Work out the finished part from the listing and answer in its coordinate system (mm). A direction names the side the tool comes from. Give positions to 0.01 mm unless a question says otherwise; leave off trailing zeros. Write each loop counter-clockwise with the first axis right and the second up, starting at its lowest first coordinate (ties: lowest second). Pieces come first, ordered by that corner, then holes. Notation, with made-up numbers: (68, 88) - (99, 88) arc R28 ccw to (99, 127) - close; hole circle Ø2 at (51, 48.25). An arc over 180 degrees is marked (long way). Write item = value, one per line.
from build123d import *

# Parameters (mm, degrees)
PAD046_DEPTH    = 9
CHAMFER016_SIZE = 3
SKETCH088_R     = 0.6
POCKET040_DEPTH = 7
SKETCH089_W     = 60.467484
SKETCH089_H     = 1.984499
PAD047_DEPTH    = 2


with BuildPart() as part:
    # Sketch085 → Pad046 (new body)
    with BuildSketch(Plane.XY.offset(-11)):
        Polygon((-30.27, -16.85), (30.27, -16.85), (30.27, -36.310793), (25.241268, -47.527155), (24.231199, -56.751064), (-24.231199, -56.751064), (-25.241268, -47.527155), (-30.27, -36.310793), align=None)
    extrude(amount=-PAD046_DEPTH)

    # Chamfer016
    chamfer016_edges = [part.edges().sort_by_distance(p)[0] for p in [
        (24.736234, -52.139109, -20),
        (27.755634, -41.918974, -20),
        (30.27, -26.580397, -20),
        (0, -16.85, -20),
        (-30.27, -26.580397, -20),
        (-27.755634, -41.918974, -20),
        (-24.736234, -52.139109, -20),
    ]]
    chamfer(chamfer016_edges, length=CHAMFER016_SIZE)

    # Sketch088 (on Face4 of Chamfer016) → Pocket040 (cut)
    with BuildSketch(Plane.XY.offset(-11)):
        with Locations((-28.523069, -29.038105)):
            Circle(SKETCH088_R)
        with Locations((28.50172, -29.085497)):
            Circle(SKETCH088_R)
        with Locations((20.999411, -47.657658)):
            Circle(SKETCH088_R)
        with Locations((-21.032127, -47.690895)):
            Circle(SKETCH088_R)
        Polygon((-28.906572, -18.901762), (28.906572, -18.901762), (28.906572, -26.491486), (26.18985, -26.491486), (26.18985, -31.415663), (28.906572, -31.415663), (23.726078, -46.130531), (19.745981, -45.128311), (18.640522, -50.078386), (18.640522, -55.110878), (-18.640522, -55.110878), (-18.640522, -50.078386), (-19.745981, -45.128311), (-23.726078, -46.130531), (-28.906572, -31.415663), (-26.18985, -31.415663), (-26.18985, -26.491486), (-28.906572, -26.491486), align=None)
    extrude(amount=-POCKET040_DEPTH, mode=Mode.SUBTRACT)

    # Sketch089 (on Face4 of Pocket040) → Pad047 (join)
    with BuildSketch(Plane.XY.offset(-11)):
        with Locations((0, -17.897196)):
            Rectangle(SKETCH089_W, SKETCH089_H)
    extrude(amount=PAD047_DEPTH)


with BuildPart() as part_1:
    # Body009 placement: moved
    add(part.part.moved(Location((0, 0, -0.2))))


solid = part_1.part
1. A tool of negligible diameter and unlimited length cuts with its end or side. For faces 1 (the flat face through (0, -55.111, -15)), 2 (the flat face through (0, -18.889, -10)), 3 (the flat face through (0, -16.905, -10)), from which of +Z, -Z, +X, -X, +Y, -Y can it reach the whole face along a straight path? Write none if from no direction.
Solution:
face_1 = +Z
face_2 = +Z, +X, -X, -Y
face_3 = +Z, +X, -X, +Y
2. For a pull along Y with two mould halves and no side action, classify faces 4 (the flat face through (28.75, -26.44, -18.72)), 5 (the flat face through (-21.708, -45.622, -14.651)), 6 (the flat face through (0, -56.751, -16)) as pulls with the +Y half, pulls with the -Y half, needs draft (parallel to the pull), parting line crosses it, or undercut.
Solution:
face_4 = needs draft
face_5 = undercut
face_6 = pulls with the -Y half
3. Straight lines are drawn through the part: line 1 (Y direction, x = -6, z = -14.5); line 2 (X direction, y = -25.5, z = -15.25). For each, find the intervals that lie inside material, in ascending order.
Solution:
line_1 = -56.75 to -55.11, -18.9 to -16.85
line_2 = -30.27 to -28.91, 28.91 to 30.27
4. Given pin 1 (3 mm diameter, centred on y = -51.5, z = -18, fed in from +X); pin 2 (6 mm diameter, centred on y = -46.5, z = -12, fed in from +X); pin 3 (0.6 mm diameter, centred on y = -18, z = -10, fed in from -X), each flat-ended and moving along its own axis, determine where each tip first touches the part or whether it passes through.
Solution:
pin_1 = 24.95
pin_2 = 27.05
pin_3 = -30.23
5. Find section D-D, the plane y = -51.5. Give the vertices of the cut face in (x, z), then the cut area to 3 significant figures.
Solution:
outline = (-24.81, -17.2) - (-21.79, -20.2) - (21.79, -20.2) - (24.81, -17.2) - (24.81, -11.2) - (18.64, -11.2) - (18.64, -18.2) - (-18.64, -18.2) - (-18.64, -11.2) - (-24.81, -11.2) - close
area = 176 mm^2
6. Find section B-B, the plane y = -24. Give the vertices of the cut face in (x, z), then the cut area to 3 significant figures.
Solution:
outline = (-30.27, -17.2) - (-27.27, -20.2) - (27.27, -20.2) - (30.27, -17.2) - (30.27, -11.2) - (28.91, -11.2) - (28.91, -18.2) - (-28.91, -18.2) - (-28.91, -11.2) - (-30.27, -11.2) - close
area = 131 mm^2
7. Find section A-A, the plane z = -12.25. Give the number of separate pieces and of enclosed holes in the cut face, then the cut area to 3 significant figures.
Solution:
separate_pieces = 1
enclosed_holes = 5
area = 447 mm^2
